from build123d import *

# Parameters (mm, degrees)
SKETCH1_R                      = 6.05
SKETCH1_R_2                    = 3.05
BOSS_EXTRUDE1_DEPTH            = 10
SKETCH2_R                      = 17.5
BOSS_EXTRUDE2_DEPTH            = 6.5
CUT_EXTRUDE1_REACH             = 28.693
SKETCH3_R                      = 2.2
CUT_EXTRUDE2_DEPTH             = 30.744747435
CUT_EXTRUDE2_DEPTH_BACK        = 30.744747435
SKETCH4_R                      = 1.5
CUT_EXTRUDE3_REACH             = 28.693
SKETCH6_R                      = 3.125
CUT_EXTRUDE3_DIRECTION_2_REACH = 28.693


with BuildPart() as part:
    # Sketch1 → Boss-Extrude1 (new body)
    with BuildSketch(Plane(origin=(0, 0, 0), x_dir=(1, 0, 0), z_dir=(0, 1, 0))):
        with Locations(Location((0, 0, 0), (0, 0, 270))):
            Circle(SKETCH1_R)
        with Locations(Location((0, 0, 0), (0, 0, 270))):
            Circle(SKETCH1_R_2, mode=Mode.SUBTRACT)
    extrude(amount=BOSS_EXTRUDE1_DEPTH)

    # Sketch2 → Boss-Extrude2 (add)
    with BuildSketch(Plane(origin=(0, 10, 0), x_dir=(1, 0, 0), z_dir=(0, 1, 0))):
        with Locations(Location((0, 0, 0), (0, 0, 90))):
            Circle(SKETCH2_R)
    extrude(amount=BOSS_EXTRUDE2_DEPTH)

    # Sketch3 → Cut-Extrude1 (cut, up to next)
    with BuildSketch(Plane.XZ.offset(-10), mode=Mode.PRIVATE) as cut_extrude1_sk1:
        with Locations(Location((12, 0, 0), (0, 0, 270))):
            Circle(SKETCH3_R)
    cut_extrude1_tool1 = extrude(cut_extrude1_sk1.sketch, amount=-CUT_EXTRUDE1_REACH, mode=Mode.PRIVATE) & part.part
    # Sketch3 → Cut-Extrude1 (cut, up to next)
    with BuildSketch(Plane.XZ.offset(-10), mode=Mode.PRIVATE) as cut_extrude1_sk2:
        with Locations(Location((0, -12, 0), (0, 0, 270))):
            Circle(SKETCH3_R)
    cut_extrude1_tool2 = extrude(cut_extrude1_sk2.sketch, amount=-CUT_EXTRUDE1_REACH, mode=Mode.PRIVATE) & part.part
    # Sketch3 → Cut-Extrude1 (cut, up to next)
    with BuildSketch(Plane.XZ.offset(-10), mode=Mode.PRIVATE) as cut_extrude1_sk3:
        with Locations(Location((-12, 0, 0), (0, 0, 270))):
            Circle(SKETCH3_R)
    cut_extrude1_tool3 = extrude(cut_extrude1_sk3.sketch, amount=-CUT_EXTRUDE1_REACH, mode=Mode.PRIVATE) & part.part
    # Sketch3 → Cut-Extrude1 (cut, up to next)
    with BuildSketch(Plane.XZ.offset(-10), mode=Mode.PRIVATE) as cut_extrude1_sk4:
        with Locations(Location((0, 12, 0), (0, 0, 270))):
            Circle(SKETCH3_R)
    cut_extrude1_tool4 = extrude(cut_extrude1_sk4.sketch, amount=-CUT_EXTRUDE1_REACH, mode=Mode.PRIVATE) & part.part
    add(cut_extrude1_tool1.solids().sort_by_distance((12, 10, 0))[0], mode=Mode.SUBTRACT)
    add(cut_extrude1_tool2.solids().sort_by_distance((0, 10, -12))[0], mode=Mode.SUBTRACT)
    add(cut_extrude1_tool3.solids().sort_by_distance((-12, 10, 0))[0], mode=Mode.SUBTRACT)
    add(cut_extrude1_tool4.solids().sort_by_distance((0, 10, 12))[0], mode=Mode.SUBTRACT)

    # Sketch4 → Cut-Extrude2 (cut, two sides: drawn at the far end of the back side and taken through both)
    with BuildSketch(Plane(origin=(0, 0, 0), x_dir=(0, 0, -1), z_dir=(1, 0, 0)).offset(-CUT_EXTRUDE2_DEPTH_BACK)):
        with Locations((0, 4.916404418)):
            Circle(SKETCH4_R)
    extrude(amount=CUT_EXTRUDE2_DEPTH + CUT_EXTRUDE2_DEPTH_BACK, mode=Mode.SUBTRACT)

    # Sketch6 → Cut-Extrude3 (cut, up to next)
    with BuildSketch(Plane(origin=(0, 10, 0), x_dir=(-1, 0, 0), z_dir=(0, -1, 0)), mode=Mode.PRIVATE) as cut_extrude3_sk1:
        with Locations(Location((0, 0, 0), (0, 0, 270))):
            Circle(SKETCH6_R)
    cut_extrude3_tool1 = extrude(cut_extrude3_sk1.sketch, amount=-CUT_EXTRUDE3_REACH, mode=Mode.PRIVATE) & part.part
    add(cut_extrude3_tool1.solids().sort_by_distance((0, 10, 0))[0], mode=Mode.SUBTRACT)

    # Sketch6 → Cut-Extrude3 direction 2 (cut, up to next)
    with BuildSketch(Plane(origin=(0, 10, 0), x_dir=(-1, 0, 0), z_dir=(0, -1, 0)), mode=Mode.PRIVATE) as cut_extrude3_direction_2_sk1:
        with Locations(Location((0, 0, 0), (0, 0, 270))):
            Circle(SKETCH6_R)
    cut_extrude3_direction_2_tool1 = extrude(cut_extrude3_direction_2_sk1.sketch, amount=CUT_EXTRUDE3_DIRECTION_2_REACH, mode=Mode.PRIVATE) & part.part
    add(cut_extrude3_direction_2_tool1.solids().sort_by_distance((0, 10, 0))[0], mode=Mode.SUBTRACT)


solid = part.part
For this review, take the finished solid that the model builds, in its own axes (mm). A direction names the side the tool comes from. Round coordinates to 2 decimals unless told otherwise and drop trailing zeros. Order: outer loops, then holes, each group sorted by start corner. A loop starts at its lowest first (then second) coordinate and runs counter-clockwise, first axis right, second up. Notation, with made-up numbers: (3, 84) -> (40, 84) arc R15 cw to (40, 103) -> close; hole circle Ø4 at (60.25, -6). An arc over 180 degrees is marked (long way). Write item = value, one per line. Start each with the question number.
1) Take a section at B-B on x = 0. State the section outline as (y, z) points (3 decimals).
2) Take a section at A-A on z = 0. State the section outline as (x, y) points (3 decimals), plus the area to 3 significant figures.
3) Take a section at D-D on z = 12. State the section outline as (x, y) points.
4) Take a section at C-C on y = 5.75. State the section outline as (x, z) points (3 decimals).
5) Tool access review of faces 1 (the face through (8, 10, 0)), 2 (the face through (-4.42, 4.98, 1.5)): name each direction out of +Z, -Z, +X, -X, +Y, -Y from which nothing blocks a thin tool from reaching the whole face with its end or side.
6) Insertion check: pin 1 (5 mm diameter, centred on y = 4.92, z = 0, fed in from +X); pin 2 (8 mm diameter, centred on x = 8, y = 11.5, fed in from -Z); pin 3 (4 mm diameter, centred on x = 0, z = 0, fed in from -Y); pin 4 (2 mm diameter, centred on x = 9.5, z = 2, fed in from -Y). Each pin has a flat end and moves straight along its axis. Give the tip position at first contact, or say it passes through.
7) To check wall thickness, follow line 1 (Y direction, x = -4.5, z = 0); line 2 (Z direction, x = -0.5, y = 11.25); line 3 (Y direction, x = 5.5, z = -7). State the ranges of each line that lie inside material, in increasing order. Write a range as from..to.
8) The part is to be moulded in two halves that separate along X. For faces 3 (the face through (2.772, 8.134, 1.442)), 4 (the face through (-3, 0, 3)), 5 (the face through (10.648, 13.204, 13.887)), say which applies: +X half, -X half, draft (parallel to the pull), parting line (faces both ways), or undercut.
Verdict:
q1.outline = (0, -6.05) -> (10, -6.05) -> (10, -9.8) -> (16.5, -9.8) -> (16.5, -3.125) -> (0, -3.125) -> close; (0, 3.125) -> (16.5, 3.125) -> (16.5, 9.8) -> (10, 9.8) -> (10, 6.05) -> (0, 6.05) -> close; (10, -17.5) -> (16.5, -17.5) -> (16.5, -14.2) -> (10, -14.2) -> close; (10, 14.2) -> (16.5, 14.2) -> (16.5, 17.5) -> (10, 17.5) -> close
q2.outline = (-17.5, 10) -> (-14.2, 10) -> (-14.2, 16.5) -> (-17.5, 16.5) -> close; (-9.8, 10) -> (-6.05, 10) -> (-6.05, 6.416) -> (-3.125, 6.416) -> (-3.125, 16.5) -> (-9.8, 16.5) -> close; (-6.05, 0) -> (-3.125, 0) -> (-3.125, 3.416) -> (-6.05, 3.416) -> close; (3.125, 0) -> (6.05, 0) -> (6.05, 3.416) -> (3.125, 3.416) -> close; (3.125, 6.416) -> (6.05, 6.416) -> (6.05, 10) -> (9.8, 10) -> (9.8, 16.5) -> (3.125, 16.5) -> close; (14.2, 10) -> (17.5, 10) -> (17.5, 16.5) -> (14.2, 16.5) -> close
q2.area = 171 mm2
q3.outline = (-12.74, 10) -> (-2.2, 10) -> (-2.2, 16.5) -> (-12.74, 16.5) -> close; (2.2, 10) -> (12.74, 10) -> (12.74, 16.5) -> (2.2, 16.5) -> close
q4.outline = (-5.92, -1.247) arc R6.05 ccw to (5.92, -1.247) -> (2.865, -1.247) arc R3.125 cw to (-2.865, -1.247) -> close; (-5.92, 1.247) -> (-2.865, 1.247) arc R3.125 cw to (2.865, 1.247) -> (5.92, 1.247) arc R6.05 ccw to start
q5.face_1 = -Y
q5.face_2 = +X, -X
q6.pin_1 = 6.05
q6.pin_2 = -17.04
q6.pin_3 = through
q6.pin_4 = 10
q7.line_1 = 0..3.42, 6.42..16.5
q7.line_2 = -17.49..-14.14, -9.86..-3.08, 3.08..9.86, 14.14..17.49
q7.line_3 = 10..16.5
q8.face_3 = undercut
q8.face_4 = draft
q8.face_5 = parting line
